```python
from build123d import *

# Parameters (mm, degrees)
F0_R     = 2.926405
F1_DEPTH = 4


with BuildPart() as f1:
    # F0 (on Front) → F1 (new body)
    with BuildSketch(Plane.XZ):
        with BuildLine():
            ThreePointArc((0, 6.35), (1.859872, 1.859872), (6.35, 0))
            Line((6.35, 0), (132.85, 0))
            ThreePointArc((132.85, 0), (137.340128, 1.859872), (139.2, 6.35))
            ThreePointArc((139.2, 6.35), (137.340128, 10.840128), (132.85, 12.7))
            Line((132.85, 12.7), (6.35, 12.7))
            ThreePointArc((6.35, 12.7), (1.859872, 10.840128), (0, 6.35))
        make_face()
        with Locations((6.35, 6.35)):
            Circle(F0_R, mode=Mode.SUBTRACT)
        with Locations((19, 6.35)):
            Circle(F0_R, mode=Mode.SUBTRACT)
        with Locations((31.65, 6.35)):
            Circle(F0_R, mode=Mode.SUBTRACT)
        with Locations((44.3, 6.35)):
            Circle(F0_R, mode=Mode.SUBTRACT)
        with Locations((56.95, 6.35)):
            Circle(F0_R, mode=Mode.SUBTRACT)
        with Locations((69.6, 6.35)):
            Circle(F0_R, mode=Mode.SUBTRACT)
        with Locations((82.25, 6.35)):
            Circle(F0_R, mode=Mode.SUBTRACT)
        with Locations((94.9, 6.35)):
            Circle(F0_R, mode=Mode.SUBTRACT)
        with Locations((107.55, 6.35)):
            Circle(F0_R, mode=Mode.SUBTRACT)
        with Locations((120.2, 6.35)):
            Circle(F0_R, mode=Mode.SUBTRACT)
        with Locations((132.85, 6.35)):
            Circle(F0_R, mode=Mode.SUBTRACT)
    extrude(amount=F1_DEPTH)


solid = f1.part
```
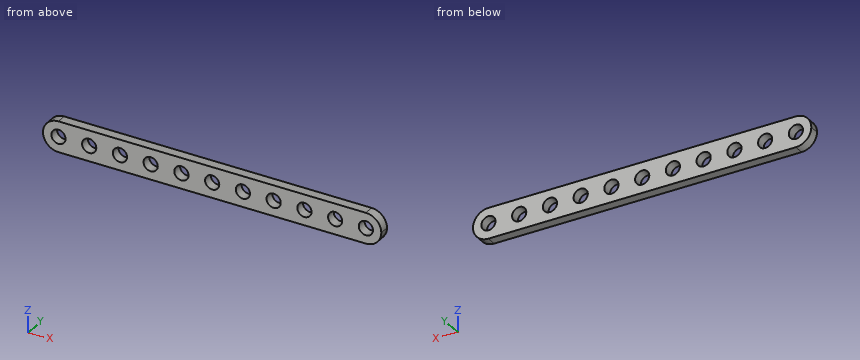
Geometry check sheet. Reference: the model listing, model coordinates, mm. Coordinates: 2 decimals unless noted, no trailing zeros. Loops run counter-clockwise (first coordinate to the right, second up) from the corner with the lowest first, then second, coordinate; pieces in that order, holes last. Notation, with made-up numbers: (77, 8) -> (90, 8) arc R26 cw to (90, 25) -> close; hole circle Ø8 at (14, 89). An arc over 180 degrees is marked (long way). Put each result on its own line as item: value.
1) Gauge pin test, flat ends, axial feed: pin 1 Ø1 at (y, z) = (-2.5, 4.5) entering from -X; pin 2 Ø3.5 at (x, z) = (132.85, 6.35) entering from +Y. Record the tip position at first contact, or that the pin passes through.
Result set:
pin 1: stops at x = 0.15
pin 2: passes through
2) Thickness scan on line 1 (Z direction, x = 56.95, y = -1.15); line 2 (Z direction, x = 69, y = -1.25); line 3 (X direction, y = -1.5, z = 11.25). Record the ranges inside material, lowest first.
Result set:
line 1: z = 0 to 3.42, 9.28 to 12.7
line 2: z = 0 to 3.49, 9.21 to 12.7
line 3: x = 2.31 to 136.89
3) Cross-section at A-A on x = 107.55. Record the boundary of the cut face in (y, z).
Result set:
outline: (-4, 0) -> (0, 0) -> (0, 3.42) -> (-4, 3.42) -> close; (-4, 9.28) -> (0, 9.28) -> (0, 12.7) -> (-4, 12.7) -> close
4) Cross-section at D-D on x = 56.5. Record the boundary of the cut face in (y, z), plus the area to 3 significant figures.
Result set:
outline: (-4, 0) -> (0, 0) -> (0, 3.46) -> (-4, 3.46) -> close; (-4, 9.24) -> (0, 9.24) -> (0, 12.7) -> (-4, 12.7) -> close
area: 27.7 mm^2
5) Cross-section at B-B on y = -2.6. Count the separate pieces of the cut face and the enclosed holes in it, plus the area to 3 significant figures.
Result set:
separate pieces: 1
enclosed holes: 11
area: 1,440 mm^2
